The model under review builds one solid part; all positions refer to its coordinate system, in mm. A direction names the side the tool comes from. Round coordinates to 2 decimals unless told otherwise and drop trailing zeros. Loops run counter-clockwise (first coordinate to the right, second up) from the corner with the lowest first, then second, coordinate; pieces in that order, holes last. Notation, with made-up numbers: M -2,76 L 32,76 A25 ccw 32,97 Z; hole C 15,31.25 d10. An arc over 180 degrees is marked long. One line per question, with ' | ' between items.
from build123d import *

# Parameters (mm, degrees)
EXTRUDE_2_DEPTH     = 5
SKETCH_5_R          = 6
CUT_EXTRUDE_2_DEPTH = 15
FILLET_1_R          = 10
FILLET_2_R          = 10
FILLET_3_R          = 10
FILLET_6_R          = 10
FILLET_8_R          = 2.5


with BuildPart() as part:
    # 草图2 → 凸台-拉伸2 (new body)
    with BuildSketch(Plane(origin=(0, 0, 0), x_dir=(1, 0, 0), z_dir=(0, 1, 0))):
        Polygon((0, 0), (19.954469714, 0), (19.954469714, -100.254623121), (-36.614072781, -156.823165616), (-63.639610307, -163.639610307), (0, -100), align=None)
    extrude(amount=EXTRUDE_2_DEPTH)

    # 草图5 → 切除-拉伸2 (cut)
    with BuildSketch(Plane(origin=(0, 5, 0), x_dir=(1, 0, 0), z_dir=(0, 1, 0))):
        with Locations(Location((9.977234857, -15, 0), (0, 0, 270))):
            Circle(SKETCH_5_R)
        with Locations(Location((9.977234857, -35, 0), (0, 0, 270))):
            Circle(SKETCH_5_R)
    extrude(amount=-CUT_EXTRUDE_2_DEPTH, mode=Mode.SUBTRACT)

    # 圆角1
    fillet_1_edges = [part.edges().sort_by_distance(p)[0] for p in [
        (0, 2.5, 100),
    ]]
    fillet(fillet_1_edges, radius=FILLET_1_R)

    # 圆角2
    fillet_2_edges = [part.edges().sort_by_distance(p)[0] for p in [
        (19.954469714, 2.5, 100.254623121),
    ]]
    fillet(fillet_2_edges, radius=FILLET_2_R)

    # 圆角3
    fillet_3_edges = [part.edges().sort_by_distance(p)[0] for p in [
        (-36.614072781, 2.5, 156.823165616),
    ]]
    fillet(fillet_3_edges, radius=FILLET_3_R)

    # 圆角6
    fillet_6_edges = [part.edges().sort_by_distance(p)[0] for p in [
        (0, 2.5, 0),
    ]]
    fillet(fillet_6_edges, radius=FILLET_6_R)

    # 圆角8
    fillet_8_edges = [part.edges().sort_by_distance(p)[0] for p in [
        (-51.464251164, 5, 160.568712564),
        (19.954469714, 0, 48.056243749),
        (19.954469714, 5, 48.056243749),
        (19.193265039, 5, 99.939321821),
        (-8.818959374, 0, 129.02805221),
        (-8.818959374, 5, 129.02805221),
        (-36.79844273, 5, 156.498325602),
        (-51.464251164, 0, 160.568712564),
    ]]
    fillet(fillet_8_edges, radius=FILLET_8_R - 0.0001)  # a hair under: the kernel refuses the full size


solid = part.part
1) Insertion check: P1, Ø2, axis at y = 1.5, z = 140.5, coming from the +X side; P2, Ø3, axis at y = 3.5, z = 52.5, coming from the -X side; P3, Ø3, axis at x = 6, y = 1.5, coming from the -Z side. Each pin has a flat end and moves straight along its axis. Give the tip position at first contact, or say it passes through.
Output values:
P1: stops at x = -19.48 | P2: stops at x = 0 | P3: stops at z = 0.32
2) For line 1 (X direction, y = 2.45, z = 15); line 2 (Z direction, x = 15.5, y = 3.2) (3 decimals); line 3 (Z direction, x = 10, y = 2.15), list the stretches that pass through material, from the lowest coordinate up.
Output values:
line 1: x = 0 to 3.98, 15.98 to 19.95 | line 2: z = 0 to 12.655, 17.345 to 32.655, 37.345 to 104.568 | line 3: z = 0 to 9, 21 to 29, 41 to 110.17
3) Add section B-B on y = 1. State the section outline as (x, z) points.
Output values:
outline: M -62.95,162.95 L -2.93,102.93 A10 cw 0,95.86 L 0,10 A10 ccw 10,0 L 19.45,0 L 19.45,96.11 A9.5 ccw 16.67,102.83 L -35.02,154.52 A9.5 ccw -39.41,157.01 Z; hole C 9.98,15 d12; hole C 9.98,35 d12
4) Machinability: for faces 1 (the flat face through (0, 2, 54)), 2 (the flat face through (2, 5, 80)), which of the approach directions +Z, -Z, +X, -X, +Y, -Y give a long, thin tool a straight path to every point of the face, cutting with its end or side? Answer none if there is none.
Output values:
face 1: -Z, -X, +Y, -Y | face 2: +Z, -Z, +X, -X, +Y
